```python
from build123d import *

# Parameters (mm, degrees)
SKETCH_1_R                      = 15
EXTRUDE_1_DEPTH                 = 30
EXTRUDE_3_DEPTH                 = 5
SKETCH_6_W                      = 5
SKETCH_6_H                      = 30
EXTRUDE_4_DEPTH                 = 30
RIB_START                       = -2.5
RIB_3_DEPTH                     = 5
PATTERN_CIRCULAR_1_COUNT        = 2
PATTERN_CIRCULAR_1_ANGLE        = 90
PATTERN_START                   = -2.5
PATTERN_CIRCULAR_1_COPY_1_DEPTH = 5
CUT_EXTRUDE_1_DEPTH             = 25
SKETCH_9_R                      = 8.5
CUT_EXTRUDE_3_DEPTH             = 42.231056256
EXTRUDE_START                   = 25
SKETCH_10_R                     = 5
SKETCH_10_R_2                   = 2
EXTRUDE_5_DEPTH                 = 5
SKETCH_10_2_R                   = 2
CUT_EXTRUDE_4_DEPTH             = 42.231056256
FILLET_1_R                      = 10


# Read off the part's stored shape, not the designer's step: 筋3
with BuildPart() as part:
    # 草图1 → 凸台-拉伸1 (new body)
    with BuildSketch(Plane.XY):
        Circle(SKETCH_1_R)
    extrude(amount=EXTRUDE_1_DEPTH)

    # 草图3 → 凸台-拉伸3 (add)
    with BuildSketch(Plane.XY.offset(30)):
        Polygon((20, -8.284271247), (20, 8.284271247), (8.284271247, 20), (-8.284271247, 20), (-20, 8.284271247), (-20, -8.284271247), (-8.284271247, -20), (8.284271247, -20), align=None)
    extrude(amount=-EXTRUDE_3_DEPTH)

    # 草图6 → 凸台-拉伸4 (add, through all)
    with BuildSketch(Plane.XY):
        Rectangle(SKETCH_6_W, SKETCH_6_H)
    extrude_4 = extrude(amount=EXTRUDE_4_DEPTH)

    # 筋3 outline → 筋3 (add)
    with BuildSketch(Plane(origin=(0, 0, 0), x_dir=(0, 0, -1), z_dir=(1, 0, 0)).offset(RIB_START)):
        Polygon((0, 15), (-19, 20), (-25, 20), (-25, 15), align=None)
    rib_3 = extrude(amount=RIB_3_DEPTH)

    # 镜向1: 筋3 across plane
    add(rib_3.mirror(Plane.ZX))

    # 阵列(圆周)1: 凸台-拉伸4, 筋3 ×2 about axis
    pattern_circular_1_axis = Axis((0, 0, 0), (0, 0, 1))
    add([extrude_4.rotate(pattern_circular_1_axis, i * PATTERN_CIRCULAR_1_ANGLE / (PATTERN_CIRCULAR_1_COUNT - 1)) for i in range(1, PATTERN_CIRCULAR_1_COUNT)])
    add([rib_3.rotate(pattern_circular_1_axis, i * PATTERN_CIRCULAR_1_ANGLE / (PATTERN_CIRCULAR_1_COUNT - 1)) for i in range(1, PATTERN_CIRCULAR_1_COUNT)])

    # 阵列(圆周)1 copy 1 sketch → 阵列(圆周)1 copy 1 (add)
    with BuildSketch(Plane(origin=(0, 0, 0), x_dir=(0, 0, -1), z_dir=(0, 1, 0)).offset(PATTERN_START)):
        Polygon((0, -15), (-19, -20), (-25, -20), (-25, -15), align=None)
    extrude(amount=PATTERN_CIRCULAR_1_COPY_1_DEPTH)

    # 草图8 → 切除-拉伸1 (cut)
    with BuildSketch(Plane.XY.offset(30)):
        Polygon((6.92820323, 12), (-6.92820323, 12), (-13.856406461, 0), (-6.92820323, -12), (6.92820323, -12), (13.856406461, 0), align=None)
    extrude(amount=-CUT_EXTRUDE_1_DEPTH, mode=Mode.SUBTRACT)

    # 草图9 → 切除-拉伸3 (cut, through all)
    with BuildSketch(Plane.XY):
        Circle(SKETCH_9_R)
    extrude(amount=CUT_EXTRUDE_3_DEPTH, mode=Mode.SUBTRACT)

    # 草图10 → 凸台-拉伸5 (add, through all)
    # profile 1 of 4: a face of its own
    with BuildSketch(Plane.XY.offset(EXTRUDE_START)):
        with Locations((14.142135624, 14.142135624)):
            Circle(SKETCH_10_R)
        with Locations((14.142135624, 14.142135624)):
            Circle(SKETCH_10_R_2, mode=Mode.SUBTRACT)
    # profile 2 of 4: a face of its own
    with BuildSketch(Plane.XY.offset(EXTRUDE_START)):
        with Locations((14.142135624, -14.142135624)):
            Circle(SKETCH_10_R)
        with Locations((14.142135624, -14.142135624)):
            Circle(SKETCH_10_R_2, mode=Mode.SUBTRACT)
    # profile 3 of 4: a face of its own
    with BuildSketch(Plane.XY.offset(EXTRUDE_START)):
        with Locations((-14.142135624, -14.142135624)):
            Circle(SKETCH_10_R)
        with Locations((-14.142135624, -14.142135624)):
            Circle(SKETCH_10_R_2, mode=Mode.SUBTRACT)
    # profile 4 of 4: a face of its own
    with BuildSketch(Plane.XY.offset(EXTRUDE_START)):
        with Locations((-14.142135624, 14.142135624)):
            Circle(SKETCH_10_R)
        with Locations((-14.142135624, 14.142135624)):
            Circle(SKETCH_10_R_2, mode=Mode.SUBTRACT)
    extrude(amount=EXTRUDE_5_DEPTH)

    # 草图10<2> → 切除-拉伸4 (cut, through all)
    with BuildSketch(Plane.XY):
        with Locations((-14.142135624, 14.142135624)):
            Circle(SKETCH_10_2_R)
        with Locations((14.142135624, 14.142135624)):
            Circle(SKETCH_10_2_R)
        with Locations((14.142135624, -14.142135624)):
            Circle(SKETCH_10_2_R)
        with Locations((-14.142135624, -14.142135624)):
            Circle(SKETCH_10_2_R)
    extrude(amount=CUT_EXTRUDE_4_DEPTH, mode=Mode.SUBTRACT)

    # 圆角1
    # the kernel refuses this fillet: 10 mm, written as the material it adds along each edge
    with BuildSketch(Plane(origin=(10.606601718, -17.67766953, 30), x_dir=(0.9019133199255954, -0.4319170792418269, 0), z_dir=(0, 0, -1)), Plane(origin=(17.67766953, 10.606601718, 30), x_dir=(0.43191707924182504, 0.9019133199255963, 0), z_dir=(0, 0, -1)), Plane(origin=(-10.606601718, 17.67766953, 30), x_dir=(-0.9019133199255949, 0.4319170792418281, 0), z_dir=(0, 0, -1)), Plane(origin=(-17.67766953, -10.606601718, 30), x_dir=(-0.43191707924182854, -0.9019133199255946, 0), z_dir=(0, 0, -1))) as fillet_1_piece_1:
        with BuildLine():
            CenterArc((6.646750578, 9.431605202), FILLET_1_R, 219.30149192, 31.287792541)
            Line((-1.091486591, 3.097594978), (-1.246251334, 2.970914774))
            ThreePointArc((-1.246251334, 2.970914774), (-0.734375399, 1.482329983), (-0.188632104, -0.066467506))
            Line((-0.188632104, -0.066467506), (0.066467506, -0.188632104))
            ThreePointArc((0.066467506, -0.188632104), (1.661687645, 0.084197399), (3.256907783, -0.188632104))
            Line((3.256907783, -0.188632104), (3.323375289, 0))
        make_face()
    extrude(amount=5)
    with BuildSketch(Plane(origin=(17.67766953, -10.606601718, 30), x_dir=(0.4319170792418248, -0.9019133199255964, 0), z_dir=(0, 0, -1))) as fillet_1_piece_2:
        with BuildLine():
            CenterArc((6.646750578, -9.431605202), FILLET_1_R, 109.410715538, 31.287792541)
            Line((-1.091486591, -3.097594978), (-1.246251334, -2.970914774))
            ThreePointArc((-1.246251334, -2.970914774), (-0.734375399, -1.482329983), (-0.188632104, 0.066467506))
            Line((-0.188632104, 0.066467506), (0.066467506, 0.188632104))
            ThreePointArc((0.066467506, 0.188632104), (1.661687645, -0.084197399), (3.256907783, 0.188632104))
            Line((3.256907783, 0.188632104), (3.323375289, 0))
        make_face()
    extrude(amount=5)
    with BuildSketch(Plane(origin=(10.606601718, 17.67766953, 30), x_dir=(-0.7071067811865472, 0.7071067811865478, 0), z_dir=(0, 0, -1)), Plane(origin=(-17.67766953, 10.606601718, 30), x_dir=(-0.7071067811865486, -0.7071067811865465, 0), z_dir=(0, 0, -1)), Plane(origin=(-10.606601718, -17.67766953, 30), x_dir=(0.7071067811865476, -0.7071067811865476, 0), z_dir=(0, 0, -1))) as fillet_1_piece_3:
        with BuildLine():
            CenterArc((6.686553006, 9.4034291), FILLET_1_R, 218.821431077, 31.287792541)
            Line((-1.104482331, 3.134476367), (-1.260303038, 3.009097312))
            ThreePointArc((-1.260303038, 3.009097312), (-0.472829503, 1.595220139), (-0.2, 0))
            Line((-0.2, 0), (0, -0.2))
            ThreePointArc((0, -0.2), (1.642135624, -0.2), (3.216225612, -0.188068582))
            Line((3.216225612, -0.188068582), (3.284271247, 0))
        make_face()
    extrude(amount=5)


solid = part.part
```
Source: CAD feature listing. Evaluate the final solid. Frame: model axes, mm. A direction names the side the tool comes from. Coordinates: 2 decimals unless noted, no trailing zeros. Write each loop counter-clockwise with the first axis right and the second up, starting at its lowest first coordinate (ties: lowest second). Pieces come first, ordered by that corner, then holes. Notation, with made-up numbers: (37.25, 79) -> (57.25, 79) arc R16 cw to (57.25, 101) -> close; hole circle Ø8 at (-22, 0). An arc over 180 degrees is marked (long way). Return JSON: item names as keys, results as strings. Group by question number.
1) Ray query, line 1 along Y through (x, z) = (6, 28.5); line 2 along Y through (x, z) = (13.5, 26.5); line 3 along Z through (x, y) = (-4, -8). Return the intervals inside material, ascending.
2) Contact query for flat-ended pins moving along their axis: P1, Ø15.5, axis at x = 0, y = 0, coming from the +Z side; P2, Ø8, axis at y = -5, z = 11.5, coming from the +X side; P3, Ø6.5, axis at x = -14.14, y = 14.14, coming from the -Z side; P4, Ø4, axis at x = 12.5, z = 21.5, coming from the -Y side. Output: stop coordinate, or through.
3) Mould query, pull axis Y, two halves, no side actions, for faces 4 (the face through (17, 2.5, 15)), 5 (the face through (19.185, -10.921, 27.535)), 6 (the face through (20, 0, 26)). Classes: +Y half, -Y half, draft (parallel to the pull), parting line (faces both ways), or undercut.
4) Section query A-A, the plane x = 0. Return loops of the section in (y, z).
5) Section query D-D, the plane z = 14. Return loops of the section in (x, y).
6) Section query B-B, the plane y = 6. Return loops of the section in (x, z), plus the area to 3 significant figures.
7) Set-up query: faces 1 (the face through (-17, -2.5, 15)), 2 (the face through (12, -13, 25)), 3 (the face through (0, -12, 18)). Return all of +Z, -Z, +X, -X, +Y, -Y with unobstructed straight access to the full face (end or side cutting, diameter ignored); none if empty.
8) Section query C-C, the plane z = 17.75. Return loops of the section in (x, y), plus the area to 3 significant figures.
From the geometry:
{
 "1": {"line 1": "-20 to -12, 12 to 20", "line 2": "-19.1 to -16.04, -12.25 to -0.62, 0.62 to 12.25, 16.04 to 19.1", "line 3": "0 to 5"},
 "2": {"P1": "through", "P2": "x = 18.85", "P3": "z = 25", "P4": "y = -10.71"},
 "3": {"face 4": "+Y half", "face 5": "undercut", "face 6": "draft"},
 "4": {"outline": "(-20, 19) -> (-15, 0) -> (-8.5, 0) -> (-8.5, 5) -> (-12, 5) -> (-12, 30) -> (-20, 30) -> close; (8.5, 0) -> (15, 0) -> (20, 19) -> (20, 30) -> (12, 30) -> (12, 5) -> (8.5, 5) -> close"},
 "5": {"outline": "(-18.68, -2.5) -> (-14.79, -2.5) arc R15 ccw to (-2.5, -14.79) -> (-2.5, -18.68) -> (2.5, -18.68) -> (2.5, -14.79) arc R15 ccw to (14.79, -2.5) -> (18.68, -2.5) -> (18.68, 2.5) -> (14.79, 2.5) arc R15 ccw to (2.5, 14.79) -> (2.5, 18.68) -> (-2.5, 18.68) -> (-2.5, 14.79) arc R15 ccw to (-14.79, 2.5) -> (-18.68, 2.5) -> close; hole (-13.86, 0) -> (-6.93, -12) -> (6.93, -12) -> (13.86, 0) -> (6.93, 12) -> (-6.93, 12) -> close"},
 "6": {"outline": "(-20, 25) -> (-13.75, 25) -> (-13.75, 0) -> (-6.02, 0) -> (-6.02, 5) -> (-10.39, 5) -> (-10.39, 30) -> (-20, 30) -> close; (6.02, 0) -> (13.75, 0) -> (13.75, 25) -> (20, 25) -> (20, 30) -> (10.39, 30) -> (10.39, 5) -> (6.02, 5) -> close", "area": "308 mm²"},
 "7": {"face 1": "-Z, -X, -Y", "face 2": "-Z, +X, -Y", "face 3": "+Z"},
 "8": {"outline": "(-19.67, -2.5) -> (-14.79, -2.5) arc R15 ccw to (-2.5, -14.79) -> (-2.5, -19.67) -> (2.5, -19.67) -> (2.5, -14.79) arc R15 ccw to (14.79, -2.5) -> (19.67, -2.5) -> (19.67, 2.5) -> (14.79, 2.5) arc R15 ccw to (2.5, 14.79) -> (2.5, 19.67) -> (-2.5, 19.67) -> (-2.5, 14.79) arc R15 ccw to (-14.79, 2.5) -> (-19.67, 2.5) -> close; hole (-13.86, 0) -> (-6.93, -12) -> (6.93, -12) -> (13.86, 0) -> (6.93, 12) -> (-6.93, 12) -> close", "area": "303 mm²"}
}
